```python
from build123d import *

# Parameters (mm, degrees)
EXTRUDE_1_DEPTH     = 60
SKETCH_2_R          = 3.3
CUT_EXTRUDE_1_DEPTH = 83.462112512
SKETCH_3_R          = 3.3
CUT_EXTRUDE_2_DEPTH = 83.462112512
FILLET_1_R          = 5
FILLET_2_R          = 3


with BuildPart() as part:
    # 草圖1 → 填料-伸長1 (new body)
    with BuildSketch(Plane(origin=(0, 0, 0), x_dir=(0, 0, -1), z_dir=(1, 0, 0))):
        Polygon((0, 0), (40, 0), (40, 6), (6, 6), (6, 40), (0, 40), align=None)
    extrude(amount=EXTRUDE_1_DEPTH)

    # 草圖2 → 除料-伸長1 (cut, through all)
    with BuildSketch(Plane(origin=(0, 0, 0), x_dir=(1, 0, 0), z_dir=(0, 1, 0))):
        with Locations(Location((10, 30, 0), (0, 0, 90))):
            Circle(SKETCH_2_R)
        with Locations(Location((50, 30, 0), (0, 0, 90))):
            Circle(SKETCH_2_R)
    extrude(amount=CUT_EXTRUDE_1_DEPTH, mode=Mode.SUBTRACT)

    # 草圖3 → 除料-伸長2 (cut, through all)
    with BuildSketch(Plane.XY):
        with Locations((10, 30)):
            Circle(SKETCH_3_R)
        with Locations((50, 30)):
            Circle(SKETCH_3_R)
    extrude(amount=-CUT_EXTRUDE_2_DEPTH, mode=Mode.SUBTRACT)

    # 圓角1
    fillet_1_edges = [part.edges().sort_by_distance(p)[0] for p in [
        (30, 6, -6),
    ]]
    fillet(fillet_1_edges, radius=FILLET_1_R)

    # 圓角2
    fillet_2_edges = [part.edges().sort_by_distance(p)[0] for p in [
        (30, 0, 0),
    ]]
    fillet(fillet_2_edges, radius=FILLET_2_R)


solid = part.part
```
Design review of the part built by this model. Coordinates are the model's own, in mm. A direction names the side the tool comes from. Round coordinates to 2 decimals unless told otherwise and drop trailing zeros. Write each loop counter-clockwise with the first axis right and the second up, starting at its lowest first coordinate (ties: lowest second). Pieces come first, ordered by that corner, then holes. Notation, with made-up numbers: (-32, 35) -> (12, 35) arc R27 ccw to (12, 68) -> close; hole circle Ø5 at (51, 18). An arc over 180 degrees is marked (long way). Answer in a Markdown table with one row per item.
Q1. Take a section at C-C, the plane x = 10. State the section outline as (y, z) points.
The answers:
| item | result |
|---|---|
| outline | (0, -40) -> (6, -40) -> (6, -33.3) -> (0, -33.3) -> close; (0, -26.7) -> (6, -26.7) -> (6, -11) arc R5 cw to (11, -6) -> (26.7, -6) -> (26.7, 0) -> (3, 0) arc R3 ccw to (0, -3) -> close; (33.3, -6) -> (40, -6) -> (40, 0) -> (33.3, 0) -> close |
Q2. Clearance check with flat-ended pins moving along their axes: pin 1 Ø3 at (x, y) = (23.5, 30) entering from +Z; pin 2 Ø3 at (x, y) = (49.5, 23) entering from -Z. State where each tip first meets the part, or that it passes through.
The answers:
| item | result |
|---|---|
| pin 1 | z = 0 |
| pin 2 | z = -6 |
Q3. To check wall thickness, follow L1, parallel to X at y = 1, z = -30; L2, parallel to Y at x = 29.5, z = -31; L3, parallel to Z at x = 49, y = 11.5. State the ranges of each line that lie inside material, in increasing order. Write a range as [from, to].
The answers:
| item | result |
|---|---|
| L1 | [0, 6.7], [13.3, 46.7], [53.3, 60] |
| L2 | [0, 6] |
| L3 | [-6, 0] |
Q4. Take a section at A-A, the plane z = -30. State the section outline as (x, y) points, then the cut area to 3 significant figures.
The answers:
| item | result |
|---|---|
| outline | (0, 0) -> (6.7, 0) -> (6.7, 6) -> (0, 6) -> close; (13.3, 0) -> (46.7, 0) -> (46.7, 6) -> (13.3, 6) -> close; (53.3, 0) -> (60, 0) -> (60, 6) -> (53.3, 6) -> close |
| area | 281 mm² |
Q5. Take a section at B-B, the plane y = 30. State the section outline as (x, z) points.
The answers:
| item | result |
|---|---|
| outline | (0, -6) -> (6.7, -6) -> (6.7, 0) -> (0, 0) -> close; (13.3, -6) -> (46.7, -6) -> (46.7, 0) -> (13.3, 0) -> close; (53.3, -6) -> (60, -6) -> (60, 0) -> (53.3, 0) -> close |
Q6. Draft analysis for pull direction Y (two halves, no side actions). For faces 3 (the face through (30, 40, -3)), 4 (the face through (30, 3, -40)), 5 (the face through (6.7, 30.1, -3)), state which applies: +Y half, -Y half, draft (parallel to the pull), parting line (faces both ways), or undercut.
The answers:
| item | result |
|---|---|
| face 3 | +Y half |
| face 4 | draft |
| face 5 | undercut |
Q7. Take a section at D-D, the plane x = 39. State the section outline as (y, z) points, then the cut area to 3 significant figures.
The answers:
| item | result |
|---|---|
| outline | (0, -40) -> (6, -40) -> (6, -11) arc R5 cw to (11, -6) -> (40, -6) -> (40, 0) -> (3, 0) arc R3 ccw to (0, -3) -> close |
| area | 447 mm² |
Q8. For faces 1 (the face through (30, 6, -26)), 2 (the face through (47.217, 2.958, -31.774)), list the 3-axis set-ups (+Z, -Z, +X, -X, +Y, -Y) from which the entire face can be reached by the end or side of a thin tool; tool diameter is ignored.
The answers:
| item | result |
|---|---|
| face 1 | -Z, +X, -X, +Y |
| face 2 | +Y, -Y |
